```python
from build123d import *

# Parameters (mm, degrees)
SKETCH_1_R      = 1
EXTRUDE_1_DEPTH = 2


with BuildPart() as part:
    # 草圖1 → 填料-伸長1 (new body)
    with BuildSketch(Plane.XY):
        with BuildLine():
            Line((-31.390669594, -5.425), (-31.390669594, -7.425))
            Line((-31.390669594, -7.425), (12.609330406, -7.425))
            Line((12.609330406, -7.425), (12.609330406, -5.425))
            ThreePointArc((12.609330406, -5.425), (11.609330406, -4.425), (12.609330406, -3.425))
            Line((12.609330406, -3.425), (14.609330406, -3.425))
            Line((14.609330406, -3.425), (14.609330406, 0.575))
            Line((14.609330406, 0.575), (12.609330406, 0.575))
            ThreePointArc((12.609330406, 0.575), (11.609330406, 1.575), (12.609330406, 2.575))
            Line((12.609330406, 2.575), (12.609330406, 4.575))
            Line((12.609330406, 4.575), (-31.390669594, 4.575))
            Line((-31.390669594, 4.575), (-31.390669594, 2.575))
            ThreePointArc((-31.390669594, 2.575), (-30.390669594, 1.575), (-31.390669594, 0.575))
            Line((-31.390669594, 0.575), (-33.390669594, 0.575))
            Line((-33.390669594, 0.575), (-33.390669594, -3.425))
            Line((-33.390669594, -3.425), (-31.390669594, -3.425))
            ThreePointArc((-31.390669594, -3.425), (-30.390669594, -4.425), (-31.390669594, -5.425))
        make_face()
        with Locations((-29.390669594, -1.425)):
            Circle(SKETCH_1_R, mode=Mode.SUBTRACT)
        with Locations((10.609330406, -1.425)):
            Circle(SKETCH_1_R, mode=Mode.SUBTRACT)
    extrude(amount=EXTRUDE_1_DEPTH)


solid = part.part
```
CAD build for the part. Positions are in the model's coordinates, mm. A direction names the side the tool comes from. Round coordinates to 2 decimals unless told otherwise and drop trailing zeros. Order: outer loops, then holes, each group sorted by start corner. A loop starts at its lowest first (then second) coordinate and runs counter-clockwise, first axis right, second up. Notation, with made-up numbers: (31.25, 60.5) - (69.25, 60.5) arc R11 cw to (69.25, 78.5) - close; hole circle Ø2 at (40.25, 25.5). An arc over 180 degrees is marked (long way). Use CSV: the item, a comma, the result in double quotes. Start each with the question number.
1) Tool access for faces 1 (the flat face through (14, -3.425, 1)), 2 (the flat face through (14, 0.575, 1)), 3 (the flat face through (-32, 0.575, 1)): list every direction of +Z, -Z, +X, -X, +Y, -Y with a clear straight run to the whole face (end or side of a thin tool).
2) Saw through at A-A (z = 0.9). List the corners of the cut face in (x, y) (3 decimals), and give its area (3 significant figures).
3) Saw through at D-D (y = 3.5). List the corners of the cut face in (x, z), and give its area (3 significant figures).
4) Two-plate mould, pull along Y, no slides. Class faces 4 (the flat face through (12.609, -6, 1)), 5 (the flat face through (-9, 4.575, 1)), 6 (the cylindrical face through (-30.39, -4.4, 0.99)): pulls with the +Y half, pulls with the -Y half, needs draft (parallel to the pull), parting line crosses it, or undercut.
5) Saw through at C-C (x = -29.5). List the corners of the cut face in (y, z) (3 decimals), and give its area (3 significant figures).
6) Pin check, flat tips, straight feed: pin 1 Ø0.6 at (y, z) = (-6, 0.5) entering from +X; pin 2 Ø0.6 at (x, z) = (-32.5, 1) entering from +Y (3 decimals); pin 3 Ø6 at (x, y) = (7.5, -5.5) entering from -Z; pin 4 Ø1 at (y, z) = (3.5, 1.5) entering from -X. Stop position of each tip, or through.
7) Wall check: L1, parallel to X at y = -2, z = 0.1; L2, parallel to X at y = 3.25, z = 1.9; L3, parallel to X at y = 1.5, z = 1.2. Give the ranges that are in metal, low to high. Write a range as [from, to].
8) Saw through at B-B (y = -1). List the corners of the cut face in (x, z), and give its area (3 significant figures).
Values follow:
1,face 1,"+Z, -Z, +X, -Y"
1,face 2,"+Z, -Z, +X, +Y"
1,face 3,"+Z, -Z, -X, +Y"
2,outline,"(-33.391, -3.425) - (-31.391, -3.425) arc R1 cw to (-31.391, -5.425) - (-31.391, -7.425) - (12.609, -7.425) - (12.609, -5.425) arc R1 cw to (12.609, -3.425) - (14.609, -3.425) - (14.609, 0.575) - (12.609, 0.575) arc R1 cw to (12.609, 2.575) - (12.609, 4.575) - (-31.391, 4.575) - (-31.391, 2.575) arc R1 cw to (-31.391, 0.575) - (-33.391, 0.575) - close; hole circle Ø2 at (-29.391, -1.425); hole circle Ø2 at (10.609, -1.425)"
2,area,"531 mm2"
3,outline,"(-31.39, 0) - (12.61, 0) - (12.61, 2) - (-31.39, 2) - close"
3,area,"88.0 mm2"
4,face 4,"needs draft"
4,face 5,"pulls with the +Y half"
4,face 6,"undercut"
5,outline,"(-7.425, 0) - (-2.419, 0) - (-2.419, 2) - (-7.425, 2) - close; (-0.431, 0) - (4.575, 0) - (4.575, 2) - (-0.431, 2) - close"
5,area,"20.0 mm2"
6,pin 1,"stops at x = 12.61"
6,pin 2,"stops at y = 0.575"
6,pin 3,"stops at z = 0"
6,pin 4,"stops at x = -31.39"
7,L1,"x = [-33.39, -30.21], [-28.57, 9.79], [11.43, 14.61]"
7,L2,"x = [-31.39, 12.61]"
7,L3,"x = [-30.39, 11.61]"
8,outline,"(-33.39, 0) - (-30.3, 0) - (-30.3, 2) - (-33.39, 2) - close; (-28.49, 0) - (9.7, 0) - (9.7, 2) - (-28.49, 2) - close; (11.51, 0) - (14.61, 0) - (14.61, 2) - (11.51, 2) - close"
8,area,"88.8 mm2"
